from build123d import *

# Parameters (mm, degrees)
F0_W     = 35
F0_H     = 2
F1_DEPTH = 34
F2_W     = 47
F2_H     = 4.5
F2_R     = 1
F3_DEPTH = 2.5
F4_R     = 0.74


with BuildPart() as f1:
    # F0 (on Top) → F1 (new body)
    with BuildSketch(Plane.XY):
        with Locations((17.5, 1)):
            Rectangle(F0_W, F0_H)
    extrude(amount=F1_DEPTH)

    # F2 (on Top) → F3 (join)
    with BuildSketch(Plane.XY):
        with Locations((17.5, 1)):
            Rectangle(F2_W, F2_H)
        with Locations((-3, 1)):
            Circle(F2_R, mode=Mode.SUBTRACT)
        with Locations((38, 1)):
            Circle(F2_R, mode=Mode.SUBTRACT)
    extrude(amount=-F3_DEPTH)

    # F4
    f4_edges = [f1.edges().sort_by_distance(p)[0] for p in [
        (-6, 1, -2.5),
        (17.5, -1.25, -2.5),
        (41, 1, -2.5),
        (17.5, 3.25, -2.5),
    ]]
    fillet(f4_edges, radius=F4_R)


solid = f1.part
Input: part model. Units: mm. Frame: model coordinates. A direction names the side the tool comes from. Coordinates: 2 decimals unless noted, no trailing zeros. Loops run counter-clockwise (first coordinate to the right, second up) from the corner with the lowest first, then second, coordinate; pieces in that order, holes last.
Q1. Cut plane A-A (y = 1). Output: boundary loops of the cut face in (x, z).
Q2. Draft query along X for faces 1 (the face through (17, 1, -2.5)), 2 (the face through (-3.8, 0.4, -1.2)), 3 (the face through (35, 1, 17)). Return one class per face: +X half, -X half, draft (parallel to the pull), parting line (faces both ways), or undercut.
Q3. Material intervals for line 1 (Y direction, x = 38, z = -1.65); line 2 (Z direction, x = 5.5, y = -0.5); line 3 (Y direction, x = 21, z = 11.5), sorted ascending.
Q4. Cut plane B-B (x = 38). Output: boundary loops of the cut face in (y, z).
Q5. Contact query for flat-ended pins moving along their axis: pin 1 (1.6 mm diameter, centred on y = 1, z = 13.5, fed in from -X); pin 2 (12 mm diameter, centred on x = 35.5, z = 18, fed in from +Y); pin 3 (2.5 mm diameter, centred on x = -3, y = 1, fed in from +Z). Output: stop coordinate, or through.
Q6. Cut plane C-C (x = 16). Output: boundary loops of the cut face in (y, z).
Q7. Set-up query: faces 4 (the face through (17, 0, 17)), 5 (the face through (17, 2, 17)), 6 (the face through (0, 1, 17)). Return all of +Z, -Z, +X, -X, +Y, -Y with unobstructed straight access to the full face (end or side cutting, diameter ignored); none if empty.
Q8. Cut plane D-D (z = 18.5). Output: boundary loops of the cut face in (x, y), then the cut area to 3 significant figures.
Working result:
1. outline: (-6, -1.76) arc R0.74 ccw to (-5.26, -2.5) - (-4, -2.5) - (-4, 0) - (-6, 0) - close; (-2, -2.5) - (37, -2.5) - (37, 0) - (35, 0) - (35, 34) - (0, 34) - (0, 0) - (-2, 0) - close; (39, -2.5) - (40.26, -2.5) arc R0.74 ccw to (41, -1.76) - (41, 0) - (39, 0) - close
2. face 1: draft
2. face 2: undercut
2. face 3: +X half
3. line 1: y = -1.25 to 0, 2 to 3.25
3. line 2: z = -2.5 to 0
3. line 3: y = 0 to 2
4. outline: (-1.25, -1.76) arc R0.74 ccw to (-0.51, -2.5) - (0, -2.5) - (0, 0) - (-1.25, 0) - close; (2, -2.5) - (2.51, -2.5) arc R0.74 ccw to (3.25, -1.76) - (3.25, 0) - (2, 0) - close
5. pin 1: stops at x = 0
5. pin 2: stops at y = 2
5. pin 3: stops at z = 0
6. outline: (-1.25, -1.76) arc R0.74 ccw to (-0.51, -2.5) - (2.51, -2.5) arc R0.74 ccw to (3.25, -1.76) - (3.25, 0) - (2, 0) - (2, 34) - (0, 34) - (0, 0) - (-1.25, 0) - close
7. face 4: +Z, +X, -X, -Y
7. face 5: +Z, +X, -X, +Y
7. face 6: +Z, -X, +Y, -Y
8. outline: (0, 0) - (35, 0) - (35, 2) - (0, 2) - close
8. area: 70.0 mm2
